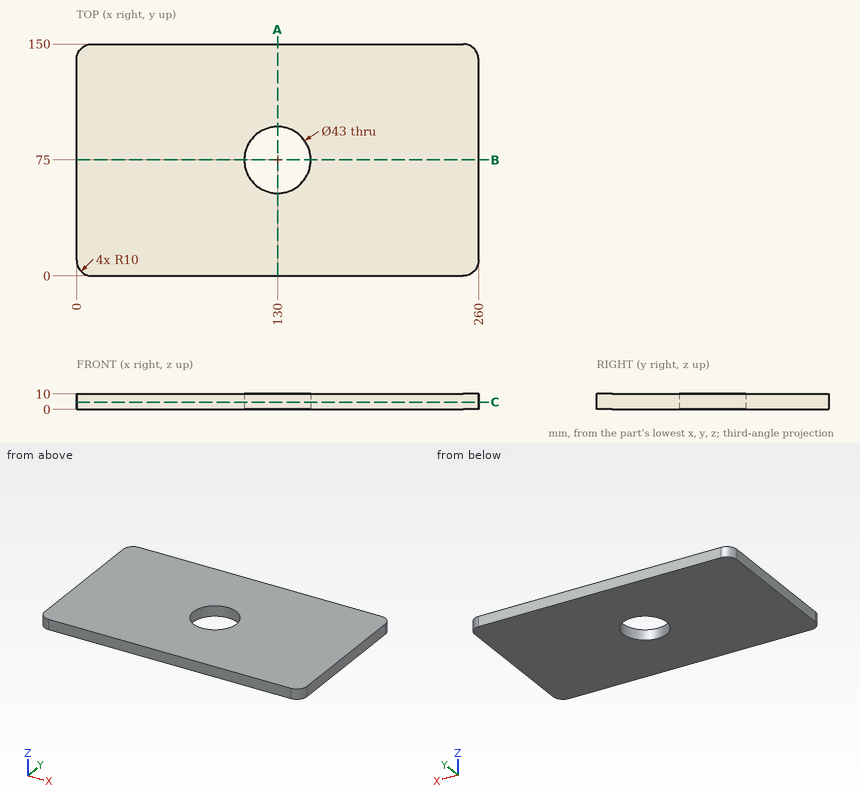
Design review of the part shown in the three views and the two pictorial views. Dimensions are in mm from the part's minimum x, y and z. Coordinates: 2 decimals unless noted, no trailing zeros. Loops run counter-clockwise (first coordinate to the right, second up) from the corner with the lowest first, then second, coordinate; pieces in that order, holes last. Notation, with made-up numbers: M 42,87.5 L 62,87.5 A23 cw 62,125.5 Z; hole C 82.25,-37.5 d9. An arc over 180 degrees is marked long. One line per question, with ' | ' between items.
(1) We need section A-A (x = 130). Give the boundary of the cut face in (y, z).
Filled in:
outline: M 0,0 L 53.5,0 L 53.5,10 L 0,10 Z; M 96.5,0 L 150,0 L 150,10 L 96.5,10 Z
(2) We need section B-B (y = 75). Give the boundary of the cut face in (x, z).
Filled in:
outline: M 0,0 L 108.5,0 L 108.5,10 L 0,10 Z; M 151.5,0 L 260,0 L 260,10 L 151.5,10 Z
(3) Wall thickness on probe 1 along Y at (x, z) = (130, 4.25); probe 2 along Y at (x, z) = (132, 9.25); probe 3 along X at (y, z) = (94, 2.75): over which ranges is each line inside the solid? List them lowest first.
Filled in:
probe 1: y = 0 to 53.5, 96.5 to 150 | probe 2: y = 0 to 53.59, 96.41 to 150 | probe 3: x = 0 to 119.94, 140.06 to 260
(4) For pin 1 Ø8 at (x, y) = (185, 88.5) entering from -Z, flat-tipped, find the tip position at first contact; note if it passes through.
Filled in:
pin 1: stops at z = 0
(5) We need section C-C (z = 4.75). Give the boundary of the cut face in (x, y).
Filled in:
outline: M 0,10 A10 ccw 10,0 L 250,0 A10 ccw 260,10 L 260,140 A10 ccw 250,150 L 10,150 A10 ccw 0,140 Z; hole C 130,75 d43
